Can you work these out from the model? Positions are in its coordinate system, mm. Face numbers are marked on the shaded views. A direction names the side the tool comes from. Give positions to 0.01 mm unless a question says otherwise; leave off trailing zeros. Loops run counter-clockwise (first coordinate to the right, second up) from the corner with the lowest first, then second, coordinate; pieces in that order, holes last. Notation, with made-up numbers: (82.5, 33) -> (95.5, 33) arc R20 ccw to (95.5, 67) -> close; hole circle Ø5 at (75, 3.25). An arc over 180 degrees is marked (long way). Return JSON: item names as keys, results as strings. Group by question number.
Q1. Suppose I cut it at C-C, the plane x = -11.5. Please give me the cut outline in (y, z), and give its area (3 significant figures).
Q2. Will these pins go through, and if not, where does the flat tip stop? pin 1 (2.5 mm diameter, centred on x = -31, z = 8.5, fed in from -Y); pin 2 (1.7 mm diameter, centred on x = 23.27, y = 12.68, fed in from +Z); pin 3 (1.6 mm diameter, centred on y = 15, z = 57, fed in from +X); pin 4 (3 mm diameter, centred on x = 20, y = 8.5, fed in from -Z).
Q3. Which directions (+Z, -Z, +X, -X, +Y, -Y) give clear straight access to the entire face, cutting with the end or side of a thin tool? Please do the marked faces 4 and 5.
Q4. I need wall thicknesses on line 1 along X through (y, z) = (3, 43); line 2 along Y through (x, z) = (9, 31); line 3 along X through (y, z) = (5.5, 34). Which ranges of each line are inside material? Lowest first, please. Write a range as [from, to].
Q5. Thinking about a two-plate mould opening in Z: for the marked faces 1, 2 and 3, which applies, pulls with the +Z half, pulls with the -Z half, needs draft (parallel to the pull), parting line crosses it, or undercut?
Q6. Suppose I cut it at A-A, the plane y = 6.5. Please give me the cut outline in (x, z).
Q7. Suppose I cut it at D-D, the plane z = 21.5. Please give me the cut outline in (x, y), and give its area (3 significant figures).
Q8. Suppose I cut it at B-B, the plane z = 46.5. Please give me the cut outline in (x, y).
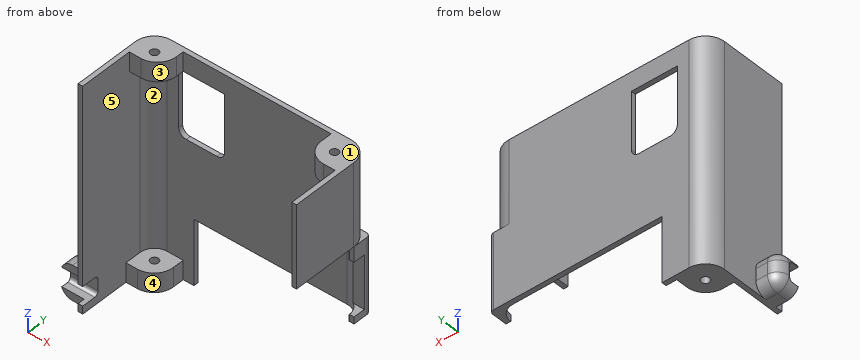
```python
from build123d import *

# Parameters (mm, degrees)
SKETCH1_W           = 57
SKETCH1_H           = 22.6
BOSS_EXTRUDE1_DEPTH = 58.4
FILLET1_R           = 5
CUT_EXTRUDE1_DEPTH  = 58.4
SKETCH3_W           = 36.8
SKETCH3_H           = 17.7
CUT_EXTRUDE2_DEPTH  = 1.2
SKETCH5_W           = 45
SKETCH5_H           = 17
CUT_EXTRUDE5_DEPTH  = 69.895242719
SKETCH6_W           = 12
SKETCH6_H           = 17
CUT_EXTRUDE6_DEPTH  = 1.2
FILLET3_R           = 2
SKETCH7_R           = 1.05
BOSS_EXTRUDE2_DEPTH = 5
FILLET4_R           = 5
BOSS_EXTRUDE3_START = -5
SKETCH8_R           = 1.05
BOSS_EXTRUDE3_DEPTH = 5
FILLET5_R           = 5
SKETCH10_W          = 9.1
SKETCH10_H          = 6
BOSS_EXTRUDE4_DEPTH = 6
CUT_EXTRUDE8_REACH  = 89.705
SKETCH11_W          = 5
SKETCH11_H          = 5
FILLET6_R           = 3
FILLET7_R           = 3
FILLET8_R           = 1
SKETCH12_W          = 57
SKETCH12_H          = 0.4
CUT_EXTRUDE9_DEPTH  = 71.208070265
BOSS_EXTRUDE5_DEPTH = 19.8
SKETCH4_W           = 14
SKETCH4_H           = 3.2
CUT_EXTRUDE3_DEPTH  = 5
FILLET9_R           = 1


with BuildPart() as part:
    # Sketch1 → Boss-Extrude1 (new body)
    with BuildSketch(Plane.XY):
        with Locations((-0.22689453, 6.382078673)):
            Rectangle(SKETCH1_W, SKETCH1_H)
    extrude(amount=BOSS_EXTRUDE1_DEPTH)

    # Fillet1
    fillet1_edges = [part.edges().sort_by_distance(p)[0] for p in [
        (-28.72689453, 17.682078673, 29.2),
        (28.27310547, 17.682078673, 29.2),
    ]]
    fillet(fillet1_edges, radius=FILLET1_R)

    # Sketch2 → Cut-Extrude1 (cut)
    with BuildSketch(Plane.XY.offset(58.4)):
        with BuildLine():
            Line((-27.52689453, -4.917921327), (27.07310547, -4.917921327))
            Line((27.07310547, -4.917921327), (27.07310547, 12.682078673))
            ThreePointArc((27.07310547, 12.682078673), (25.960111239, 15.369084441), (23.27310547, 16.482078673))
            Line((23.27310547, 16.482078673), (-23.72689453, 16.482078673))
            ThreePointArc((-23.72689453, 16.482078673), (-26.413900298, 15.369084441), (-27.52689453, 12.682078673))
            Line((-27.52689453, 12.682078673), (-27.52689453, -4.917921327))
        make_face()
    extrude(amount=-CUT_EXTRUDE1_DEPTH, mode=Mode.SUBTRACT)

    # Sketch3 → Cut-Extrude2 (cut)
    with BuildSketch(Plane(origin=(28.27310547, 0, 0), x_dir=(0, 0, -1), z_dir=(1, 0, 0))):
        with Locations((-18.4, 3.932078673)):
            Rectangle(SKETCH3_W, SKETCH3_H)
    extrude(amount=-CUT_EXTRUDE2_DEPTH, mode=Mode.SUBTRACT)

    # Sketch5 → Cut-Extrude5 (cut, through all)
    with BuildSketch(Plane(origin=(0, 17.682078673, 0), x_dir=(1, 0, 0), z_dir=(0, 1, 0))):
        with Locations((5.77210537, -8.5)):
            Rectangle(SKETCH5_W, SKETCH5_H)
    extrude(amount=-CUT_EXTRUDE5_DEPTH, mode=Mode.SUBTRACT)

    # Sketch6 → Cut-Extrude6 (cut)
    with BuildSketch(Plane(origin=(0, 17.682078673, 0), x_dir=(1, 0, 0), z_dir=(0, 1, 0))):
        with Locations((-14.72689453, -44.9)):
            Rectangle(SKETCH6_W, SKETCH6_H)
    extrude(amount=-CUT_EXTRUDE6_DEPTH, mode=Mode.SUBTRACT)

    # Fillet3
    fillet3_edges = [part.edges().sort_by_distance(p)[0] for p in [
        (-20.72689453, 17.082078673, 36.4),
        (-8.72689453, 17.082078673, 36.4),
    ]]
    fillet(fillet3_edges, radius=FILLET3_R)

    # Sketch7 → Boss-Extrude2 (add)
    # profile 1 of 2: a face of its own
    with BuildSketch(Plane.XY.offset(58.4)):
        with BuildLine():
            Line((-27.52689453, 9.482078673), (-19.52689453, 9.482078673))
            Line((-19.52689453, 9.482078673), (-19.52689453, 16.482078673))
            Line((-19.52689453, 16.482078673), (-23.72689453, 16.482078673))
            ThreePointArc((-23.72689453, 16.482078673), (-26.413900298, 15.369084441), (-27.52689453, 12.682078673))
            Line((-27.52689453, 12.682078673), (-27.52689453, 9.482078673))
        make_face()
        with Locations((-23.72689453, 12.682078673)):
            Circle(SKETCH7_R, mode=Mode.SUBTRACT)
    # profile 2 of 2: a face of its own
    with BuildSketch(Plane.XY.offset(58.4)):
        with BuildLine():
            Line((19.07310547, 16.482078673), (19.07310547, 8.482078673))
            Line((19.07310547, 8.482078673), (27.07310547, 8.482078673))
            Line((27.07310547, 8.482078673), (27.07310547, 12.682078673))
            ThreePointArc((27.07310547, 12.682078673), (25.960111239, 15.369084441), (23.27310547, 16.482078673))
            Line((23.27310547, 16.482078673), (19.07310547, 16.482078673))
        make_face()
        with Locations((23.27310547, 12.682078673)):
            Circle(SKETCH7_R, mode=Mode.SUBTRACT)
    extrude(amount=-BOSS_EXTRUDE2_DEPTH)

    # Fillet4
    fillet4_edges = [part.edges().sort_by_distance(p)[0] for p in [
        (-19.52689453, 9.482078673, 55.9),
        (19.07310547, 8.482078673, 55.9),
    ]]
    fillet(fillet4_edges, radius=FILLET4_R)

    # Sketch8 → Boss-Extrude3 (add)
    with BuildSketch(Plane(origin=(0, 0, 0), x_dir=(-1, 0, 0), z_dir=(0, 0, -1)).offset(BOSS_EXTRUDE3_START)):
        with BuildLine():
            Line((19.52689453, 16.482078673), (19.52689453, 8.482078673))
            Line((19.52689453, 8.482078673), (27.52689453, 8.482078673))
            Line((27.52689453, 8.482078673), (27.52689453, 12.682078673))
            ThreePointArc((27.52689453, 12.682078673), (26.413900298, 15.369084441), (23.72689453, 16.482078673))
            Line((23.72689453, 16.482078673), (19.52689453, 16.482078673))
        make_face()
        with Locations(Location((23.72689453, 12.682078673, 0), (0, 0, 180))):
            Circle(SKETCH8_R, mode=Mode.SUBTRACT)
    extrude(amount=BOSS_EXTRUDE3_DEPTH)

    # Fillet5
    fillet5_edges = [part.edges().sort_by_distance(p)[0] for p in [
        (-19.52689453, 8.482078673, 2.5),
    ]]
    fillet(fillet5_edges, radius=FILLET5_R)

    # Sketch10 → Boss-Extrude4 (add)
    with BuildSketch(Plane.ZY.offset(28.72689453)):
        with Locations((4.55, 0.282078673)):
            Rectangle(SKETCH10_W, SKETCH10_H)
    extrude(amount=BOSS_EXTRUDE4_DEPTH)

    # Cut-Extrude8: up to this face of the body (flat: up to its plane)
    cut_extrude8_end = Plane(part.part.faces().sort_by_distance((-27.52689453, 3.623812959, 29.334734165))[0])
    # Sketch11 → Cut-Extrude8 (cut, up to the picked face)
    with BuildSketch(Plane.ZY.offset(34.72689453), mode=Mode.PRIVATE) as cut_extrude8_sk1:
        with Locations((4.55, -2.417921327)):
            Rectangle(SKETCH11_W, SKETCH11_H)
    cut_extrude8_tool1 = split(extrude(cut_extrude8_sk1.sketch, amount=-CUT_EXTRUDE8_REACH, mode=Mode.PRIVATE), bisect_by=cut_extrude8_end, keep=Keep.BOTH, mode=Mode.PRIVATE)
    add(cut_extrude8_tool1.solids().sort_by(Axis((-34.726895, -2.417921, 4.55), (1, 0, 0)))[0], mode=Mode.SUBTRACT)

    # Fillet6
    fillet6_edges = [part.edges().sort_by_distance(p)[0] for p in [
        (-31.72689453, 3.282078673, 0),
        (-31.72689453, 3.282078673, 9.1),
    ]]
    fillet(fillet6_edges, radius=FILLET6_R)

    # Fillet7
    fillet7_edges = [part.edges().sort_by_distance(p)[0] for p in [
        (-34.72689453, -1.217921327, 9.1),
        (-34.72689453, 2.403399016, 8.221320344),
        (-34.72689453, -1.217921327, 0),
        (-34.72689453, 2.403399016, 0.878679656),
        (-34.72689453, 3.282078673, 4.55),
    ]]
    fillet(fillet7_edges, radius=FILLET7_R)

    # Fillet8
    fillet8_edges = [part.edges().sort_by_distance(p)[0] for p in [
        (-31.049699857, 0.082078673, 7.05),
        (-31.049699857, 0.082078673, 2.05),
    ]]
    fillet(fillet8_edges, radius=FILLET8_R)

    # Sketch12 → Cut-Extrude9 (cut, through all)
    with BuildSketch(Plane.XY.offset(58.4)):
        with Locations((-0.22689453, -4.717921327)):
            Rectangle(SKETCH12_W, SKETCH12_H)
    extrude(amount=-CUT_EXTRUDE9_DEPTH, mode=Mode.SUBTRACT)

    # Sketch15 → Boss-Extrude5 (add)
    with BuildSketch(Plane(origin=(0, 0, 17), x_dir=(-1, 0, 0), z_dir=(0, 0, -1))):
        with BuildLine():
            Line((-28.27210537, 12.782078673), (-27.27310547, 12.782078673))
            ThreePointArc((-27.27310547, 12.782078673), (-26.101532595, 15.610505797), (-23.27310547, 16.782078673))
            Line((-23.27310547, 16.782078673), (-23.27310547, 17.682078673))
            Line((-23.27310547, 17.682078673), (-28.27210537, 17.682078673))
            Line((-28.27210537, 17.682078673), (-28.27210537, 12.782078673))
        make_face()
    extrude(amount=-BOSS_EXTRUDE5_DEPTH)

    # Sketch4 → Cut-Extrude3 (cut)
    with BuildSketch(Plane(origin=(28.27310547, 0, 0), x_dir=(0, 0, -1), z_dir=(1, 0, 0))):
        with Locations((-25.8, 14.282078673)):
            Rectangle(SKETCH4_W, SKETCH4_H)
    extrude(amount=-CUT_EXTRUDE3_DEPTH, mode=Mode.SUBTRACT)

    # Fillet9
    fillet9_edges = [part.edges().sort_by_distance(p)[0] for p in [
        (28.27210537, 17.682078673, 26.9),
    ]]
    fillet(fillet9_edges, radius=FILLET9_R)


solid = part.part
```
Ans:
{
 "1": {"outline": "(16.48, 17) -> (17.68, 17) -> (17.68, 36.4) -> (16.48, 36.4) -> close; (16.48, 53.4) -> (17.68, 53.4) -> (17.68, 58.4) -> (16.48, 58.4) -> close", "area": "29.3 mm^2"},
 "2": {"pin 1": "stops at y = -2.72", "pin 2": "passes through", "pin 3": "stops at x = 28.04", "pin 4": "stops at z = 53.4"},
 "3": {"face 4": "+Z, -Z, +X, -Y", "face 5": "-Y"},
 "4": {"line 1": "x = [-28.73, -27.53], [27.07, 28.27]", "line 2": "y = [16.48, 17.68]", "line 3": "x = [-28.73, -27.53]"},
 "5": {"face 1": "pulls with the +Z half", "face 2": "undercut", "face 3": "needs draft"},
 "6": {"outline": "(-28.73, 0) -> (-27.53, 0) -> (-27.53, 58.4) -> (-28.73, 58.4) -> close; (27.07, 36.8) -> (28.27, 36.8) -> (28.27, 58.4) -> (27.07, 58.4) -> close"},
 "7": {"outline": "(-28.73, -4.52) -> (-27.53, -4.52) -> (-27.53, 12.68) arc R3.8 cw to (-23.73, 16.48) -> (23.27, 16.48) arc R3.8 cw to (25.32, 15.88) -> (28.27, 15.88) -> (28.27, 16.68) arc R1 ccw to (27.27, 17.68) -> (-23.73, 17.68) arc R5 ccw to (-28.73, 12.68) -> close", "area": "93.3 mm^2"},
 "8": {"outline": "(-28.73, -4.52) -> (-27.53, -4.52) -> (-27.53, 12.68) arc R3.8 cw to (-23.73, 16.48) -> (-20.73, 16.48) -> (-20.73, 17.68) -> (-23.73, 17.68) arc R5 ccw to (-28.73, 12.68) -> close; (-8.73, 16.48) -> (23.27, 16.48) arc R3.8 cw to (27.07, 12.68) -> (27.07, -4.52) -> (28.27, -4.52) -> (28.27, 12.68) arc R5 ccw to (23.27, 17.68) -> (-8.73, 17.68) -> close"}
}
